```python
from build123d import *

# Parameters (mm, degrees)
SKETCH1_W             = 70
SKETCH1_H             = 40
BOSS_EXTRUDE1_DEPTH   = 3
F_3_0MM_DOWEL_HOLE1_D = 3
F_4_CLEARANCE_HOLE1_D = 3.2639
FILLET1_R             = 2


with BuildPart() as part:
    # Sketch1 → Boss-Extrude1 (new body)
    with BuildSketch(Plane(origin=(0, 0, 0), x_dir=(1, 0, 0), z_dir=(0, 1, 0))):
        Rectangle(SKETCH1_W, SKETCH1_H)
    extrude(amount=BOSS_EXTRUDE1_DEPTH)

    # Ø3.0mm Dowel Hole1 (through all)
    with Locations(Plane(origin=(0, 3, 0), x_dir=(1, 0, 0), z_dir=(0, 1, 0))):
        with Locations((-2.15, 13.9), (25.95, 13.9), (-2.15, -13.9), (25.95, -13.9)):
            Hole(F_3_0MM_DOWEL_HOLE1_D / 2)

    # #4 Clearance Hole1 (through all)
    with Locations(Plane(origin=(0, 3, 0), x_dir=(1, 0, 0), z_dir=(0, 1, 0))):
        with Locations((-31, 15), (-31, -15), (25.95, 0)):
            Hole(F_4_CLEARANCE_HOLE1_D / 2)

    # Fillet1
    fillet1_edges = [part.edges().sort_by_distance(p)[0] for p in [
        (35, 1.5, 20),
        (-35, 1.5, 20),
        (-35, 1.5, -20),
        (35, 1.5, -20),
    ]]
    fillet(fillet1_edges, radius=FILLET1_R)


solid = part.part
```
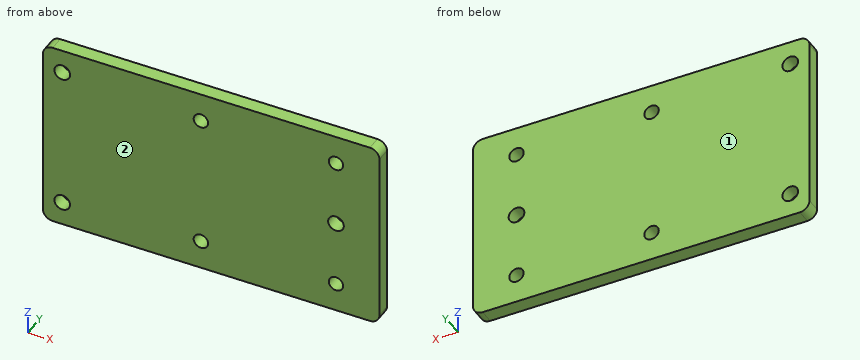
Design review of the part built by this model. Coordinates are the model's own, in mm. Face numbers are marked on the shaded views. Round coordinates to 2 decimals unless told otherwise and drop trailing zeros. Order: outer loops, then holes, each group sorted by start corner. A loop starts at its lowest first (then second) coordinate and runs counter-clockwise, first axis right, second up. Notation, with made-up numbers: (78.5, 27.25) - (128.5, 27.25) arc R24 ccw to (128.5, 46.25) - close; hole circle Ø9 at (-7, 39.25). An arc over 180 degrees is marked (long way). Return JSON: item names as keys, results as strings.
Q1. Wall thickness on L1, parallel to Z at x = -31, y = 0.75; L2, parallel to Z at x = -2.15, y = 2.1; L3, parallel to Z at x = 25.95, y = 0.7: over which ranges is each line inside the solid? List them lowest first. Write a range as [from, to].
Computed values:
{"L1": "z = [-20, -16.63], [-13.37, 13.37], [16.63, 20]", "L2": "z = [-20, -15.4], [-12.4, 12.4], [15.4, 20]", "L3": "z = [-20, -15.4], [-12.4, -1.63], [1.63, 12.4], [15.4, 20]"}
Q2. Consider section D-D on x = -31. Write out the cut boundary in (y, z), plus the area to 3 significant figures.
Computed values:
{"outline": "(0, -20) - (3, -20) - (3, -16.63) - (0, -16.63) - close; (0, -13.37) - (3, -13.37) - (3, 13.37) - (0, 13.37) - close; (0, 16.63) - (3, 16.63) - (3, 20) - (0, 20) - close", "area": "100 mm2"}
Q3. The part is to be moulded in two halves that separate along Y. For the marked faces 1 and 2, say which applies: pulls with the +Y half, pulls with the -Y half, needs draft (parallel to the pull), parting line crosses it, or undercut.
Computed values:
{"face 1": "pulls with the +Y half", "face 2": "pulls with the -Y half"}
Q4. Consider section B-B on y = 0.85. Write out the cut boundary in (x, z), plus the area to 3 significant figures.
Computed values:
{"outline": "(-35, -18) arc R2 ccw to (-33, -20) - (33, -20) arc R2 ccw to (35, -18) - (35, 18) arc R2 ccw to (33, 20) - (-33, 20) arc R2 ccw to (-35, 18) - close; hole circle Ø3.26 at (-31, -15); hole circle Ø3.26 at (-31, 15); hole circle Ø3 at (-2.15, -13.9); hole circle Ø3 at (-2.15, 13.9); hole circle Ø3.26 at (25.95, 0); hole circle Ø3 at (25.95, -13.9); hole circle Ø3 at (25.95, 13.9)", "area": "2,740 mm2"}
Q5. Consider section C-C on x = 25.95. Write out the cut boundary in (y, z), plus the area to 3 significant figures.
Computed values:
{"outline": "(0, -20) - (3, -20) - (3, -15.4) - (0, -15.4) - close; (0, -12.4) - (3, -12.4) - (3, -1.63) - (0, -1.63) - close; (0, 1.63) - (3, 1.63) - (3, 12.4) - (0, 12.4) - close; (0, 15.4) - (3, 15.4) - (3, 20) - (0, 20) - close", "area": "92.2 mm2"}
Q6. Consider section A-A on x = -2.15. Write out the cut boundary in (y, z), plus the area to 3 significant figures.
Computed values:
{"outline": "(0, -20) - (3, -20) - (3, -15.4) - (0, -15.4) - close; (0, -12.4) - (3, -12.4) - (3, 12.4) - (0, 12.4) - close; (0, 15.4) - (3, 15.4) - (3, 20) - (0, 20) - close", "area": "102 mm2"}
